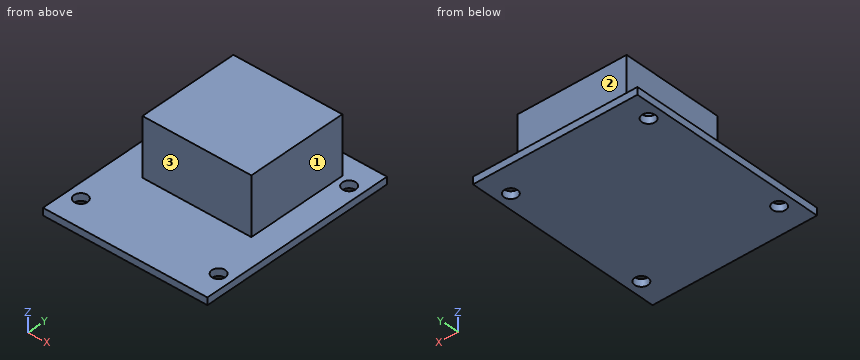
from build123d import *

# Parameters (mm, degrees)
F0_W     = 45.6
F0_H     = 55.3
F1_DEPTH = 2
F2_R     = 1.85
F3_DEPTH = 25
F4_W     = 30.2
F4_H     = 28
F5_DEPTH = 16


with BuildPart() as f1:
    # F0 (on Top) → F1 (new body)
    with BuildSketch(Plane.XY):
        Rectangle(F0_W, F0_H)
    extrude(amount=F1_DEPTH)

    # F2 (on face) → F3 (cut)
    with BuildSketch(Plane.XY.offset(2)):
        with Locations((-19.1, 20.1)):
            Circle(F2_R)
        with Locations((19.1, 20.1)):
            Circle(F2_R)
        with Locations((-19.1, -20.1)):
            Circle(F2_R)
        with Locations((19.1, -20.1)):
            Circle(F2_R)
    extrude(amount=-F3_DEPTH, mode=Mode.SUBTRACT)

    # F4 (on face) → F5 (join)
    with BuildSketch(Plane.XY.offset(2)):
        with Locations((0.7, 7.65)):
            Rectangle(F4_W, F4_H)
    extrude(amount=F5_DEPTH)


solid = f1.part
Could you check a few things on this model? Use its own coordinates, in mm. Face numbers are marked on the shaded views. A direction names the side the tool comes from. Give positions to 0.01 mm unless a question says otherwise; leave off trailing zeros. Order: outer loops, then holes, each group sorted by start corner. A loop starts at its lowest first (then second) coordinate and runs counter-clockwise, first axis right, second up. Notation, with made-up numbers: (4.5, -25.75) -> (8.5, -25.75) arc R23 cw to (8.5, -8.75) -> close; hole circle Ø10 at (36.5, 55). An arc over 180 degrees is marked (long way). Return JSON: item names as keys, results as strings.
1. For pin 1 Ø8 at (y, z) = (7.5, 10.5) entering from -X; pin 2 Ø3.5 at (x, y) = (-19.1, 20.1) entering from -Z; pin 3 Ø5 at (x, z) = (-4, 12) entering from +Y; pin 4 Ø5 at (x, z) = (-4.5, 6.5) entering from -Y, each with a flat end and sliding along its axis, tell me the tip position at first contact or that it passes through.
Answer list:
{"pin 1": "stops at x = -14.4", "pin 2": "passes through", "pin 3": "stops at y = 21.65", "pin 4": "stops at y = -6.35"}
2. I need wall thicknesses on line 1 (Y direction, x = -19.1, z = 0.8); line 2 (Z direction, x = 3, y = 25.5); line 3 (Y direction, x = -10.5, z = 16.25). Which ranges of each line are inside material? Lowest first, please. Write a range as from..to.
Answer list:
{"line 1": "y = -27.65..-21.95, -18.25..18.25, 21.95..27.65", "line 2": "z = 0..2", "line 3": "y = -6.35..21.65"}
3. Imagine slicing it at C-C on x = -5. List the corners of the cut face in (y, z) for me.
Answer list:
{"outline": "(-27.65, 0) -> (27.65, 0) -> (27.65, 2) -> (21.65, 2) -> (21.65, 18) -> (-6.35, 18) -> (-6.35, 2) -> (-27.65, 2) -> close"}
4. Imagine slicing it at B-B on x = -19.1. List the corners of the cut face in (y, z) for me.
Answer list:
{"outline": "(-27.65, 0) -> (-21.95, 0) -> (-21.95, 2) -> (-27.65, 2) -> close; (-18.25, 0) -> (18.25, 0) -> (18.25, 2) -> (-18.25, 2) -> close; (21.95, 0) -> (27.65, 0) -> (27.65, 2) -> (21.95, 2) -> close"}
5. Imagine slicing it at A-A on y = 20.1. List the corners of the cut face in (x, z) for me.
Answer list:
{"outline": "(-22.8, 0) -> (-20.95, 0) -> (-20.95, 2) -> (-22.8, 2) -> close; (-17.25, 0) -> (17.25, 0) -> (17.25, 2) -> (15.8, 2) -> (15.8, 18) -> (-14.4, 18) -> (-14.4, 2) -> (-17.25, 2) -> close; (20.95, 0) -> (22.8, 0) -> (22.8, 2) -> (20.95, 2) -> close"}
6. On a 3-axis mill with a long thin cutter (end or side, diameter ignored), from which of +Z, -Z, +X, -X, +Y, -Y can I reach the whole of each face in a straight line? I mean the marked faces 1, 2 and 3. Say none if no direction works.
Answer list:
{"face 1": "+Z, +X, +Y, -Y", "face 2": "+Z, +X, -X, +Y", "face 3": "+Z, +X, -X, -Y"}
7. Imagine slicing it at D-D on y = -24. List the corners of the cut face in (x, z) for me, then the cut area to 3 significant figures.
Answer list:
{"outline": "(-22.8, 0) -> (22.8, 0) -> (22.8, 2) -> (-22.8, 2) -> close", "area": "91.2 mm2"}
